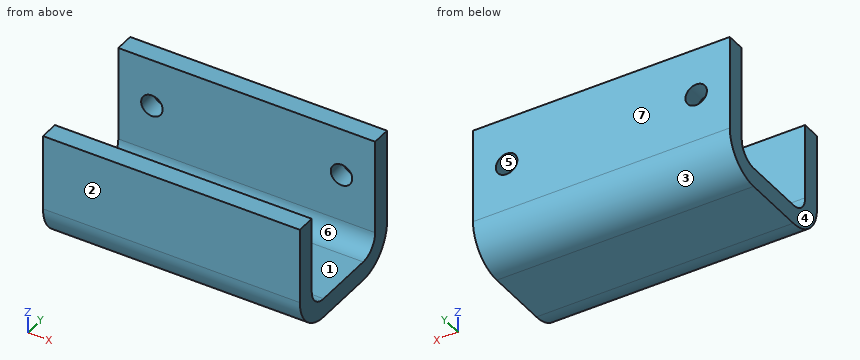
from build123d import *

# Parameters (mm, degrees)
SKETCH2_W                = 40.64
SKETCH2_H                = 15
BASE_FLANGE1_DEPTH       = 3
EDGE_FLANGE1_DEPTH       = 40.64
EDGE_FLANGE2_DEPTH       = 40.64
M3_CLEARANCE_HOLE1_D     = 3.4
M3_CLEARANCE_HOLE1_DEPTH = 3


# Sheet-metal steps are written as plain solids
with BuildPart() as part:
    # Sketch2 → Base-Flange1 (new body)
    with BuildSketch(Plane(origin=(0, 0, 0), x_dir=(1, 0, 0), z_dir=(0, 1, 0))):
        Rectangle(SKETCH2_W, SKETCH2_H)
    extrude(amount=-BASE_FLANGE1_DEPTH)

    # Edge-Flange1 section (across the edge) → Edge-Flange1 (add)
    with BuildSketch(Plane(origin=(-20.32, -3, -10.5), x_dir=(0, 0, 1), z_dir=(1, 0, 0))):
        with BuildLine():
            Line((-3, 3), (-3, 13))
            Line((-3, 13), (0, 13))
            Line((0, 13), (0, 3))
            ThreePointArc((0, 3), (0.878679656, 0.878679656), (3, 0))
            Line((3, 0), (3, -3))
            ThreePointArc((3, -3), (-1.242640687, -1.242640687), (-3, 3))
        make_face()
    extrude(amount=EDGE_FLANGE1_DEPTH)

    # Edge-Flange2 section (across the edge) → Edge-Flange2 (add)
    with BuildSketch(Plane(origin=(-20.32, -19, -10.5), x_dir=(0, 1, 0), z_dir=(1, 0, 0))):
        with BuildLine():
            Line((-3, 3), (-3, 15))
            Line((-3, 15), (0, 15))
            Line((0, 15), (0, 3))
            ThreePointArc((0, 3), (0.878679656, 0.878679656), (3, 0))
            Line((3, 0), (3, -3))
            ThreePointArc((3, -3), (-1.242640687, -1.242640687), (-3, 3))
        make_face()
    extrude(amount=EDGE_FLANGE2_DEPTH)

    # M3 Clearance Hole1
    with Locations(Plane(origin=(0, 0, 0), x_dir=(1, 0, 0), z_dir=(0, 1, 0))):
        with Locations((-15, 0), (15, 0)):
            Hole(M3_CLEARANCE_HOLE1_D / 2, depth=M3_CLEARANCE_HOLE1_DEPTH)


solid = part.part
Read the model definition and answer for the solid it produces. Units are mm, in the model's axes. Face numbers are marked on the shaded views. A direction names the side the tool comes from. Round coordinates to 2 decimals unless told otherwise and drop trailing zeros. Write each loop counter-clockwise with the first axis right and the second up, starting at its lowest first coordinate (ties: lowest second). Pieces come first, ordered by that corner, then holes.
Q1. Straight lines are drawn through the part: line 1 (Y direction, x = -7.5, z = 1); line 2 (Z direction, x = -12.5, y = -9); line 3 (Z direction, x = 15, y = -2.1). For each, find the intervals that lie inside material, in ascending order.
Values:
line 1: y = -22 to -19, -3 to 0
line 2: z = -13.5 to -10.5
line 3: z = -12.06 to -1.7, 1.7 to 7.5
Q2. Flat-ended cylindrical pins translate along their axes: P1, Ø11, axis at x = -7, y = -12.5, coming from the +Z side; P2, Ø3.5, axis at x = 0, y = -20, coming from the +Z side; P3, Ø8, axis at x = 15.5, y = -10.5, coming from the +Z side. Find the tip coordinate at first contact, or state that the pin passes through.
Values:
P1: stops at z = -9.74
P2: stops at z = 4.5
P3: stops at z = -10.5
Q3. Find section C-C on z = 0. Determine the outline of the cut face in (x, y).
Values:
outline: (-20.32, -22) - (20.32, -22) - (20.32, -19) - (-20.32, -19) - close; (-20.32, -3) - (-16.7, -3) - (-16.7, 0) - (-20.32, 0) - close; (-13.3, -3) - (13.3, -3) - (13.3, 0) - (-13.3, 0) - close; (16.7, -3) - (20.32, -3) - (20.32, 0) - (16.7, 0) - close
Q4. Find section A-A on x = -15. Determine the outline of the cut face in (y, z).
Values:
outline: (-22, -7.5) arc R6 ccw to (-16, -13.5) - (-6, -13.5) arc R6 ccw to (0, -7.5) - (0, -1.7) - (-3, -1.7) - (-3, -7.5) arc R3 cw to (-6, -10.5) - (-16, -10.5) arc R3 cw to (-19, -7.5) - (-19, 4.5) - (-22, 4.5) - close; (-3, 1.7) - (0, 1.7) - (0, 7.5) - (-3, 7.5) - close
Q5. A tool of negligible diameter and unlimited length cuts with its end or side. For the marked faces 5, 6 and 7, from which of +Z, -Z, +X, -X, +Y, -Y can it reach the whole face along a straight path? Write none if from no direction.
Values:
face 5: +Y
face 6: +Z, +X, -X
face 7: +Z, -Z, +X, -X, +Y
Q6. Find section D-D on x = 6. Determine the outline of the cut face in (y, z).
Values:
outline: (-22, -7.5) arc R6 ccw to (-16, -13.5) - (-6, -13.5) arc R6 ccw to (0, -7.5) - (0, 7.5) - (-3, 7.5) - (-3, -7.5) arc R3 cw to (-6, -10.5) - (-16, -10.5) arc R3 cw to (-19, -7.5) - (-19, 4.5) - (-22, 4.5) - close
Q7. The mould has two halves that part along Y. Classify the marked faces 1, 2, 3 and 4: released by +Y, released by -Y, zero draft, split by the parting line, or undercut.
Values:
face 1: undercut
face 2: released by -Y
face 3: released by +Y
face 4: zero draft
Q8. Find section B-B on z = -4. Determine the outline of the cut face in (x, y), and give its area (3 significant figures).
Values:
outline: (-20.32, -22) - (20.32, -22) - (20.32, -19) - (-20.32, -19) - close; (-20.32, -3) - (20.32, -3) - (20.32, 0) - (-20.32, 0) - close
area: 244 mm2
